CAD build for the part. Positions are in the model's coordinates, mm. A direction names the side the tool comes from. Coordinates: 2 decimals unless noted, no trailing zeros. Loops run counter-clockwise (first coordinate to the right, second up) from the corner with the lowest first, then second, coordinate; pieces in that order, holes last. Notation, with made-up numbers: (78, 9.25) -> (90, 9.25) arc R18 ccw to (90, 26.25) -> close; hole circle Ø2 at (-10, -3). An arc over 180 degrees is marked (long way). Answer as CSV lines item,"result". Start each with the question number.
```python
from build123d import *

# Parameters (mm, degrees)
SKETCH1_R             = 50.575792326
SKETCH1_R_2           = 2.54
BOSS_EXTRUDE1_DEPTH   = 6.35
SKETCH2_W             = 7.62
SKETCH2_H             = 5.08
SKETCH2_W_2           = 6.35
BOSS_EXTRUDE3_DEPTH   = 9.525
SKETCH3_W             = 13.97
SKETCH3_H             = 5.08
CUT_EXTRUDE1_DEPTH    = 3.175
CIRPATTERN2_START     = 6.35
CIRPATTERN2_OUTLINE_W = 9.525
CIRPATTERN2_OUTLINE_H = 13.97
CIRPATTERN2_DEPTH     = 5.08
SKETCH4_W             = 13.97
SKETCH4_H             = 5.08
CUT_EXTRUDE2_DEPTH    = 3.175


# Read off the part's stored shape, not the designer's step: CirPattern2
with BuildPart() as part:
    # Sketch1 → Boss-Extrude1 (new body)
    with BuildSketch(Plane(origin=(0, 0, 0), x_dir=(1, 0, 0), z_dir=(0, 1, 0))):
        with Locations(Location((0, 0, 0), (0, 0, 270))):
            Circle(SKETCH1_R)
        with Locations(Location((0, 0, 0), (0, 0, 270))):
            Circle(SKETCH1_R_2, mode=Mode.SUBTRACT)
    extrude(amount=BOSS_EXTRUDE1_DEPTH)

    # Sketch2 → Boss-Extrude3 (add)
    with BuildSketch(Plane(origin=(0, 0, 0), x_dir=(0, 0, -1), z_dir=(1, 0, 0))):
        with Locations((-44.218352, 8.89)):
            Rectangle(SKETCH2_W, SKETCH2_H)
        with Locations((-37.233352, 8.89)):
            Rectangle(SKETCH2_W_2, SKETCH2_H)
    extrude(amount=-BOSS_EXTRUDE3_DEPTH)

    # Sketch3 → Cut-Extrude1 (cut)
    with BuildSketch(Plane(origin=(0, 0, 0), x_dir=(0, 0, -1), z_dir=(1, 0, 0))):
        with Locations((-41.043352, 8.89)):
            Rectangle(SKETCH3_W, SKETCH3_H)
    extrude(amount=-CUT_EXTRUDE1_DEPTH, mode=Mode.SUBTRACT)

    # CirPattern2 outline → CirPattern2 (add)
    with BuildSketch(Plane(origin=(0, 0, 0), x_dir=(1, 0, 0), z_dir=(0, 1, 0)).offset(CIRPATTERN2_START)):
        with Locations((4.7625, 41.043352)):
            Rectangle(CIRPATTERN2_OUTLINE_W, CIRPATTERN2_OUTLINE_H)
    extrude(amount=CIRPATTERN2_DEPTH)

    # Sketch4 → Cut-Extrude2 (cut)
    with BuildSketch(Plane.ZY):
        with Locations((-41.043352, 8.89)):
            Rectangle(SKETCH4_W, SKETCH4_H)
    extrude(amount=-CUT_EXTRUDE2_DEPTH, mode=Mode.SUBTRACT)


solid = part.part
```
Q1. Two-plate mould, pull along X, no slides. Class faces 1 (the flat face through (6, 11.43, -41)), 2 (the flat face through (3.175, 9, -41)), 3 (the cylindrical face through (2.52, 3.13, -0.33)): pulls with the +X half, pulls with the -X half, needs draft (parallel to the pull), parting line crosses it, or undercut.
Q2. Which spindle directions (+Z, -Z, +X, -X, +Y, -Y) get a long thin tool onto all of the face, cutting with end or side? Do faces 4 (the flat face through (6, 9, -48.028)), 5 (the flat face through (-9.525, 9, 41)), 6 (the flat face through (-6, 9, 48.028)). Say none if no direction does.
Q3. Saw through at D-D (x = -14). List the corners of the cut face in (y, z), and give its area (3 significant figures).
Q4. Probe probe 1 along X at (y, z) = (5, 0); probe 2 along Y at (x, z) = (42, 9.5); probe 3 along Z at (x, y) = (0.5, 5.5). List the from-to ranges inside material, lowest first. Write a range as from..to.
Q5. Saw through at A-A (z = 0). List the corners of the cut face in (x, y), and give its area (3 significant figures).
Q6. Saw through at C-C (z = -39). List the corners of the cut face in (x, y) (3 decimals), and give its area (3 significant figures).
Q7. Saw through at B-B (x = 0). List the corners of the cut face in (y, z).
Q8. Pin check, flat tips, straight feed: pin 1 Ø5.5 at (x, y) = (5, 9.5) entering from -Z; pin 2 Ø6 at (x, y) = (8.5, 3) entering from -Z; pin 3 Ø1.5 at (y, z) = (10, 39) entering from -X (3 decimals); pin 4 Ø1 at (y, z) = (7.5, 30) entering from +X. Stop position of each tip, or through.
Ans:
1,face 1,"needs draft"
1,face 2,"pulls with the -X half"
1,face 3,"undercut"
2,face 4,"-Z, +X, -X, +Y"
2,face 5,"+Z, -Z, -X, +Y"
2,face 6,"+Z, +X, -X, +Y"
3,outline,"(0, -48.6) -> (6.35, -48.6) -> (6.35, 48.6) -> (0, 48.6) -> close"
3,area,"617 mm²"
4,probe 1,"x = -50.58..-2.54, 2.54..50.58"
4,probe 2,"y = 0..6.35"
4,probe 3,"z = -50.57..-2.49, 2.49..50.57"
5,outline,"(-50.58, 0) -> (-2.54, 0) -> (-2.54, 6.35) -> (-50.58, 6.35) -> close; (2.54, 0) -> (50.58, 0) -> (50.58, 6.35) -> (2.54, 6.35) -> close"
5,area,"610 mm²"
6,outline,"(-32.201, 0) -> (32.201, 0) -> (32.201, 6.35) -> (9.525, 6.35) -> (9.525, 11.43) -> (3.175, 11.43) -> (3.175, 6.35) -> (-32.201, 6.35) -> close"
6,area,"441 mm²"
7,outline,"(0, -50.58) -> (6.35, -50.58) -> (6.35, -2.54) -> (0, -2.54) -> close; (0, 2.54) -> (6.35, 2.54) -> (6.35, 50.58) -> (0, 50.58) -> close"
8,pin 1,"stops at z = -48.03"
8,pin 2,"stops at z = -50.28"
8,pin 3,"stops at x = -9.525"
8,pin 4,"passes through"
